CAD build for the part. Positions are in the model's coordinates, mm. A direction names the side the tool comes from. Give positions to 0.01 mm unless a question says otherwise; leave off trailing zeros. Order: outer loops, then holes, each group sorted by start corner. A loop starts at its lowest first (then second) coordinate and runs counter-clockwise, first axis right, second up. Notation, with made-up numbers: (0.25, 44.5) -> (33.25, 44.5) arc R28 cw to (33.25, 80.5) -> close; hole circle Ø1 at (46, 31). An arc over 180 degrees is marked (long way). Use one line per item in the form item = value. Start each with the question number.
1) Drop flat-ended pins along their axis: P1, Ø12, axis at y = 30.5, z = -69, coming from the -X side; P2, Ø9.5, axis at x = 3, y = -8, coming from the -Z side; P3, Ø12, axis at y = -26.5, z = -287, coming from the -X side. Give the stop position or say it passes through.
2) Tool access for faces 1 (the face through (-3.47, 15.62, -15.99)), 2 (the face through (-33.727, 25.861, -255.91)), 3 (the face through (-10.316, 7.91, -20.944)): list every direction of +Z, -Z, +X, -X, +Y, -Y with a clear straight run to the whole face (end or side of a thin tool).
3) Cut at B-B, the plane y = -37.5. State how many separate pieces and enclosed holes the cut face has, and give its area (3 significant figures).
4) Probe line 1 (X direction, y = 0, z = -13); line 2 (X direction, y = 0, z = -279.5). List the from-to ranges inside material, lowest first.
5) Cut at A-A, the plane z = -299. Give the cut face in (x, y).
6) Mould opens along Z. For faces 4 (the face through (-10.316, 7.91, -7.395)), 5 (the face through (-1.3, -13.1, -15)), 6 (the face through (1.3, -13.1, -17)) say: pulls with the +Z half, pulls with the -Z half, needs draft (parallel to the pull), parting line crosses it, or undercut.
from build123d import *

# Parameters (mm, degrees)
F2_W     = 90.759490079
F2_H     = 30
F3_DEPTH = 50


with BuildPart() as f1:
    # F0 (on Front) → F1 (revolve)
    with BuildSketch(Plane.XZ):
        with BuildLine():
            Line((0, -349), (0, -350))
            Line((0, -350), (23.5, -350))
            ThreePointArc((23.5, -350), (37.6421356237, -344.1421356237), (43.5, -330))
            Line((43.5, -330), (43.5, -190))
            add(Edge.make_bspline(
                [(43.5, -100), (43.5136655823, -109.2677385113), (39.1523633552, -123.5841908002), (24.2069666289, -139.9270455841), (36.8772857328, -158.3450760247), (43.5142465453, -178.4930156545), (43.5, -190)],
                knots=[0, 0, 0, 0, 0.2553201748, 0.4772684921, 0.7031288482, 1, 1, 1, 1], degree=3))
            add(Edge.make_bspline(
                [(13, -25), (15.153980754, -30.004083225), (26.3990720982, -29.6995209895), (44.8019804311, -78.3531291958), (42.8678392414, -88.8611251657), (43.5, -100)],
                knots=[0, 0, 0, 0, 0.239885862, 0.6752778241, 1, 1, 1, 1], degree=3))
            Line((13, -25), (13, -17))
            Line((13, -17), (16, -17))
            Line((16, -17), (16, -15))
            Line((16, -15), (13, -15))
            Line((13, -15), (13, 0))
            Line((13, 0), (12, 0))
            Line((12, 0), (12, -1))
            Line((12, -1), (12, -25.1138266176))
            add(Edge.make_bspline(
                [(42.5, -100), (42.1580635011, -92.4746021628), (43.1338322578, -76.1216357103), (25.4300825706, -29.885728794), (13.9739168808, -30.3249489516), (12, -25.1138266176)],
                knots=[0, 0, 0, 0, 0.3254300492, 0.7613683252, 1, 1, 1, 1], degree=3))
            add(Edge.make_bspline(
                [(42.5, -190), (42.0858003199, -178.4723848104), (36.3650992329, -158.3583449355), (23.0339165178, -139.8179083613), (38.4175773884, -124.0130301912), (42.7362024784, -108.3010882139), (42.5, -100)],
                knots=[0, 0, 0, 0, 0.2965395662, 0.5226698941, 0.7450400773, 1, 1, 1, 1], degree=3))
            Line((42.5, -190), (42.5, -330))
            ThreePointArc((42.5, -330), (36.9350288425, -343.4350288425), (23.5, -349))
            Line((23.5, -349), (0, -349))
        make_face()
    revolve(axis=Axis((0, 0, -175), (0, 0, -1)))

    # F2 (on Front) → F3 (cut, symmetric)
    with BuildSketch(Plane.XZ):
        with Locations((0.3664636352, -335)):
            Rectangle(F2_W, F2_H)
    extrude(amount=F3_DEPTH, both=True, mode=Mode.SUBTRACT)


solid = f1.part
Result:
q1.P1 = -32.14
q1.P2 = -27.51
q1.P3 = -38.37
q2.face_1 = +Z
q2.face_2 = -Z
q2.face_3 = none
q3.separate_pieces = 2
q3.enclosed_holes = 1
q3.area = 1,070 mm²
q4.line_1 = -13 to -12, 12 to 13
q4.line_2 = -43.5 to -42.5, 42.5 to 43.5
q5.outline = circle Ø87 at (0, 0); hole circle Ø85 at (0, 0)
q6.face_4 = needs draft
q6.face_5 = pulls with the +Z half
q6.face_6 = undercut
